Design review of the part built by this model. Coordinates are the model's own, in mm. A direction names the side the tool comes from. Coordinates: 2 decimals unless noted, no trailing zeros. Write each loop counter-clockwise with the first axis right and the second up, starting at its lowest first coordinate (ties: lowest second). Pieces come first, ordered by that corner, then holes. Notation, with made-up numbers: (1, 58) - (21, 58) arc R21 ccw to (21, 80) - close; hole circle Ø8 at (-17.5, 30). An arc over 180 degrees is marked (long way). Use a Markdown table: item, result.
from build123d import *

# Parameters (mm, degrees)
SKETCH_1_R      = 1.75
SKETCH_1_R_2    = 1.5
EXTRUDE_1_DEPTH = 4
FILLET_1_R      = 3
EXTRUDE_2_DEPTH = 4
FILLET_2_R      = 3
FILLET_3_R      = 3


with BuildPart() as part:
    # 草图1 → 凸台-拉伸1 (new body)
    with BuildSketch(Plane.XY):
        Polygon((-7.5, 7.5), (-7.5, 53.732798972), (7.5, 53.732798972), (7.5, 7.5), (24, 7.5), (24, -7.5), (-24, -7.5), (-24, 7.5), align=None)
        with Locations((0, 40)):
            Circle(SKETCH_1_R, mode=Mode.SUBTRACT)
        with Locations((0, 20)):
            Circle(SKETCH_1_R, mode=Mode.SUBTRACT)
        with Locations((16, 0)):
            Circle(SKETCH_1_R_2, mode=Mode.SUBTRACT)
        Circle(SKETCH_1_R_2, mode=Mode.SUBTRACT)
        with Locations((-16, 0)):
            Circle(SKETCH_1_R_2, mode=Mode.SUBTRACT)
    extrude(amount=EXTRUDE_1_DEPTH)

    # 圆角1
    fillet_1_edges = [part.edges().sort_by_distance(p)[0] for p in [
        (-7.5, 53.732798972, 2),
        (7.5, 53.732798972, 2),
        (7.5, 7.5, 2),
        (24, 7.5, 2),
        (24, -7.5, 2),
        (-24, -7.5, 2),
        (-24, 7.5, 2),
        (-7.5, 7.5, 2),
    ]]
    fillet(fillet_1_edges, radius=FILLET_1_R)

    # 草图2 → 凸台-拉伸2 (add)
    with BuildSketch(Plane(origin=(0, 0, 0), x_dir=(-1, 0, 0), z_dir=(0, 0, -1))):
        Polygon((4.6, -4.836204333), (4.6, -7.5), (8.6, -7.5), (8.6, 7.5), (4.6, 7.5), align=None)
        Polygon((-4.6, -4.836204333), (-4.6, 7.5), (-8.6, 7.5), (-8.6, -7.5), (-4.6, -7.5), align=None)
    extrude(amount=EXTRUDE_2_DEPTH)

    # 圆角2
    # the kernel refuses this fillet: 3 mm, written as the material it adds along each edge
    with BuildSketch(Plane(origin=(-8.6, -7.5, 0), x_dir=(-1, 0, 0), z_dir=(0, 1, 0)), Plane(origin=(8.6, 7.5, 0), x_dir=(1, 0, 0), z_dir=(0, -1, 0))) as fillet_2_piece_1:
        with BuildLine():
            CenterArc((FILLET_2_R, -FILLET_2_R), FILLET_2_R, 90, 90)
            Line((0, -FILLET_2_R), (0, 0))
            Line((0, 0), (FILLET_2_R, 0))
        make_face()
    extrude(amount=15)

    # 圆角3
    fillet_3_edges = [part.edges().sort_by_distance(p)[0] for p in [
        (-4.6, 7.5, -2),
        (4.6, 7.5, -2),
    ]]
    fillet(fillet_3_edges, radius=FILLET_3_R)


solid = part.part
(1) For L1, parallel to Y at x = 0, z = 2.9; L2, parallel to X at y = 49, z = 2; L3, parallel to Z at x = 0, y = 24, list the stretches that pass through material, from the lowest coordinate up. Write a range as from..to.
Determined:
| item | result |
|---|---|
| L1 | -7.5..-1.5, 1.5..18.25, 21.75..38.25, 41.75..53.73 |
| L2 | -7.5..7.5 |
| L3 | 0..4 |
(2) Take a section at B-B on y = 0. Write out the cut boundary in (x, z).
Determined:
| item | result |
|---|---|
| outline | (-24, 0) - (-17.5, 0) - (-17.5, 4) - (-24, 4) - close; (-14.5, 0) - (-11.6, 0) arc R3 cw to (-8.6, -3) - (-8.6, -4) - (-4.6, -4) - (-4.6, 0) - (-1.5, 0) - (-1.5, 4) - (-14.5, 4) - close; (1.5, 0) - (4.6, 0) - (4.6, -4) - (8.6, -4) - (8.6, -3) arc R3 cw to (11.6, 0) - (14.5, 0) - (14.5, 4) - (1.5, 4) - close; (17.5, 0) - (24, 0) - (24, 4) - (17.5, 4) - close |
(3) Take a section at A-A on x = -16. Write out the cut boundary in (y, z), and give its area (3 significant figures).
Determined:
| item | result |
|---|---|
| outline | (-7.5, 0) - (-1.5, 0) - (-1.5, 4) - (-7.5, 4) - close; (1.5, 0) - (7.5, 0) - (7.5, 4) - (1.5, 4) - close |
| area | 48.0 mm2 |
(4) Draft analysis for pull direction Y (two halves, no side actions). For faces 1 (the cylindrical face through (-1.5, 0.07, 1.97)), 2 (the cylindrical face through (-6.645, 52.831, 2.028)), 3 (the cylindrical face through (-0.38, 38.29, 1.97)), 4 (the flat face through (0, 17, 4)), state which applies: +Y half, -Y half, draft (parallel to the pull), parting line (faces both ways), or undercut.
Determined:
| item | result |
|---|---|
| face 1 | undercut |
| face 2 | +Y half |
| face 3 | undercut |
| face 4 | draft |
(5) Take a section at C-C on x = 0. Write out the cut boundary in (y, z), and give its area (3 significant figures).
Determined:
| item | result |
|---|---|
| outline | (-7.5, 0) - (-1.5, 0) - (-1.5, 4) - (-7.5, 4) - close; (1.5, 0) - (18.25, 0) - (18.25, 4) - (1.5, 4) - close; (21.75, 0) - (38.25, 0) - (38.25, 4) - (21.75, 4) - close; (41.75, 0) - (53.73, 0) - (53.73, 4) - (41.75, 4) - close |
| area | 205 mm2 |
(6) Take a section at D-D on y = 40. Write out the cut boundary in (x, z).
Determined:
| item | result |
|---|---|
| outline | (-7.5, 0) - (-1.75, 0) - (-1.75, 4) - (-7.5, 4) - close; (1.75, 0) - (7.5, 0) - (7.5, 4) - (1.75, 4) - close |
(7) Machinability: for faces 5 (the cylindrical face through (5.46, 6.6, -2.03)), 6 (the flat face through (18, 0, 0)), 7 (the cylindrical face through (8.36, 8.4, 2.03)), 8 (the flat face through (-7.5, 30, 2)), 9 (the flat face through (-18, 0, 0)), which of the approach directions +Z, -Z, +X, -X, +Y, -Y give a long, thin tool a straight path to every point of the face, cutting with its end or side? Answer none if there is none.
Determined:
| item | result |
|---|---|
| face 5 | -Z, +Y |
| face 6 | -Z, +X, +Y, -Y |
| face 7 | +Z, -Z, +X, +Y |
| face 8 | +Z, -Z, -X, +Y |
| face 9 | -Z, -X, +Y, -Y |
(8) For pin 1 (0.8 mm diameter, centred on y = 0.5, z = -3.5, fed in from -X); pin 2 (4 mm diameter, centred on x = -14.5, z = -1.5, fed in from +Y); pin 3 (1.5 mm diameter, centred on x = 0.5, y = 38, fed in from -Z), all flat-tipped, find the tip position at first contact; note any pin that passes through.
Determined:
| item | result |
|---|---|
| pin 1 | x = -8.6 |
| pin 2 | y = 7.5 |
| pin 3 | z = 0 |
